Source: CAD feature listing. Evaluate the final solid. Frame: model axes, mm. Face numbers are marked on the shaded views. A direction names the side the tool comes from. Give positions to 0.01 mm unless a question says otherwise; leave off trailing zeros. Order: outer loops, then holes, each group sorted by start corner. A loop starts at its lowest first (then second) coordinate and runs counter-clockwise, first axis right, second up. Notation, with made-up numbers: (31.25, 13) -> (75.25, 13) arc R14 cw to (75.25, 24) -> close; hole circle Ø3 at (-35, 43.25). An arc over 180 degrees is marked (long way). Answer in a Markdown table with one row per item.
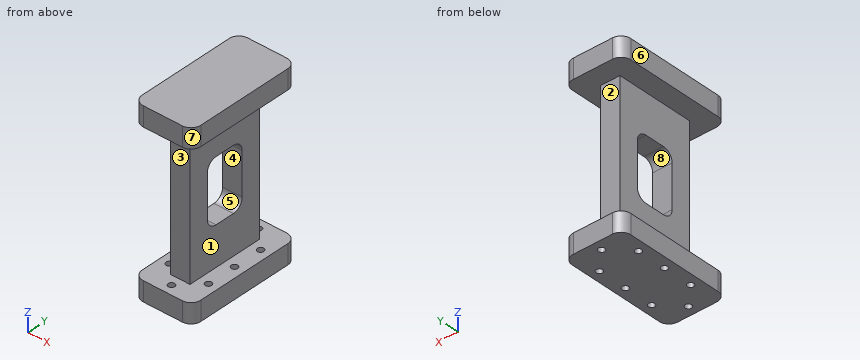
```python
from build123d import *

# Parameters (mm, degrees)
BOSS_EXTRUDE1_DEPTH       = 92
CUT_EXTRUDE1_DEPTH        = 102.311401135
CUT_EXTRUDE1_DEPTH_BACK   = 10
SKETCH3_W                 = 72
SKETCH3_H                 = 50
CUT_EXTRUDE2_DEPTH        = 10
SKETCH4_W                 = 72
SKETCH4_H                 = 10
CUT_EXTRUDE3_DEPTH        = 10
SKETCH5_W                 = 72
SKETCH5_H                 = 10
CUT_EXTRUDE4_DEPTH        = 10
M4X0_7_TAPPED_HOLE1_D     = 3.3
M4X0_7_TAPPED_HOLE1_DEPTH = 10
M4X0_7_TAPPED_HOLE2_D     = 3.3
M4X0_7_TAPPED_HOLE2_DEPTH = 10
M4X0_7_TAPPED_HOLE3_D     = 3.3
M4X0_7_TAPPED_HOLE3_DEPTH = 10
M4X0_7_TAPPED_HOLE4_D     = 3.3
M4X0_7_TAPPED_HOLE4_DEPTH = 10
M4X0_7_TAPPED_HOLE5_D     = 3.3
M4X0_7_TAPPED_HOLE5_DEPTH = 10
M4X0_7_TAPPED_HOLE6_D     = 3.3
M4X0_7_TAPPED_HOLE6_DEPTH = 10
M4X0_7_TAPPED_HOLE7_D     = 3.3
M4X0_7_TAPPED_HOLE7_DEPTH = 10
M4X0_7_TAPPED_HOLE8_D     = 3.3
M4X0_7_TAPPED_HOLE8_DEPTH = 10
CUT_EXTRUDE5_DEPTH        = 10
CUT_EXTRUDE8_DEPTH        = 10
CUT_EXTRUDE9_DEPTH        = 10


with BuildPart() as part:
    # Sketch1 → Boss-Extrude1 (new body)
    with BuildSketch(Plane.XY):
        with BuildLine():
            Line((-10, -30), (10, -30))
            ThreePointArc((10, -30), (13.535533906, -28.535533906), (15, -25))
            Line((15, -25), (15, 25))
            ThreePointArc((15, 25), (13.535533906, 28.535533906), (10, 30))
            Line((10, 30), (-10, 30))
            ThreePointArc((-10, 30), (-13.535533906, 28.535533906), (-15, 25))
            Line((-15, 25), (-15, -25))
            ThreePointArc((-15, -25), (-13.535533906, -28.535533906), (-10, -30))
        make_face()
    extrude(amount=BOSS_EXTRUDE1_DEPTH)

    # Sketch2 → Cut-Extrude1 (cut, two sides: drawn at the far end of the back side and taken through both)
    with BuildSketch(Plane(origin=(15, 0, 0), x_dir=(0, 0, -1), z_dir=(1, 0, 0)).offset(-CUT_EXTRUDE1_DEPTH_BACK)):
        Polygon((-10, 25), (-82, 25), (-82, -25), (-10, -25), (-10, 0), align=None)
    extrude(amount=CUT_EXTRUDE1_DEPTH + CUT_EXTRUDE1_DEPTH_BACK, mode=Mode.SUBTRACT)

    # Sketch3 → Cut-Extrude2 (cut)
    with BuildSketch(Plane.ZY.offset(15)):
        with Locations((46, 0)):
            Rectangle(SKETCH3_W, SKETCH3_H)
    extrude(amount=-CUT_EXTRUDE2_DEPTH, mode=Mode.SUBTRACT)

    # Sketch4 → Cut-Extrude3 (cut)
    with BuildSketch(Plane.ZY.offset(5)):
        with Locations((46, 25)):
            Rectangle(SKETCH4_W, SKETCH4_H)
    extrude(amount=-CUT_EXTRUDE3_DEPTH, mode=Mode.SUBTRACT)

    # Sketch5 → Cut-Extrude4 (cut)
    with BuildSketch(Plane.ZY.offset(5)):
        with Locations((46, -25)):
            Rectangle(SKETCH5_W, SKETCH5_H)
    extrude(amount=-CUT_EXTRUDE4_DEPTH, mode=Mode.SUBTRACT)

    # M4x0.7 Tapped Hole1
    with Locations(Plane.XY.offset(10)):
        with Locations((10, -15)):
            Hole(M4X0_7_TAPPED_HOLE1_D / 2, depth=M4X0_7_TAPPED_HOLE1_DEPTH)

    # M4x0.7 Tapped Hole2
    with Locations(Plane.XY.offset(10)):
        with Locations((10, 0)):
            Hole(M4X0_7_TAPPED_HOLE2_D / 2, depth=M4X0_7_TAPPED_HOLE2_DEPTH)

    # M4x0.7 Tapped Hole3
    with Locations(Plane.XY.offset(10)):
        with Locations((10, 15)):
            Hole(M4X0_7_TAPPED_HOLE3_D / 2, depth=M4X0_7_TAPPED_HOLE3_DEPTH)

    # M4x0.7 Tapped Hole4
    with Locations(Plane.XY.offset(10)):
        with Locations((-10, -15)):
            Hole(M4X0_7_TAPPED_HOLE4_D / 2, depth=M4X0_7_TAPPED_HOLE4_DEPTH)

    # M4x0.7 Tapped Hole5
    with Locations(Plane.XY.offset(10)):
        with Locations((-10, 0)):
            Hole(M4X0_7_TAPPED_HOLE5_D / 2, depth=M4X0_7_TAPPED_HOLE5_DEPTH)

    # M4x0.7 Tapped Hole6
    with Locations(Plane.XY.offset(10)):
        with Locations((-10, 15)):
            Hole(M4X0_7_TAPPED_HOLE6_D / 2, depth=M4X0_7_TAPPED_HOLE6_DEPTH)

    # M4x0.7 Tapped Hole7
    with Locations(Plane.XY.offset(10)):
        with Locations((0, 25)):
            Hole(M4X0_7_TAPPED_HOLE7_D / 2, depth=M4X0_7_TAPPED_HOLE7_DEPTH)

    # M4x0.7 Tapped Hole8
    with Locations(Plane.XY.offset(10)):
        with Locations((0, -25)):
            Hole(M4X0_7_TAPPED_HOLE8_D / 2, depth=M4X0_7_TAPPED_HOLE8_DEPTH)

    # Sketch27 → Cut-Extrude5 (cut)
    with BuildSketch(Plane.ZY.offset(5)):
        with BuildLine():
            Line((62, 0), (62, 5))
            ThreePointArc((62, 5), (60.535533906, 8.535533906), (57, 10))
            Line((57, 10), (35, 10))
            ThreePointArc((35, 10), (31.464466094, 8.535533906), (30, 5))
            Line((30, 5), (30, 0))
            Line((30, 0), (30, -5))
            ThreePointArc((30, -5), (31.464466094, -8.535533906), (35, -10))
            Line((35, -10), (57, -10))
            ThreePointArc((57, -10), (60.535533906, -8.535533906), (62, -5))
            Line((62, -5), (62, 0))
        make_face()
    extrude(amount=-CUT_EXTRUDE5_DEPTH, mode=Mode.SUBTRACT)

    # Sketch29 → Cut-Extrude8 (cut)
    with BuildSketch(Plane.ZY.offset(15)):
        Polygon((82, -25), (82, 25), (82, 39.435498448), (10, 39.435498448), (10, -37.130826461), (82, -37.130826461), align=None)
    extrude(amount=-CUT_EXTRUDE8_DEPTH, mode=Mode.SUBTRACT)

    # Sketch30 → Cut-Extrude9 (cut)
    with BuildSketch(Plane(origin=(15, 0, 0), x_dir=(0, 0, -1), z_dir=(1, 0, 0))):
        Polygon((-82, 25), (-82, -25), (-82, -44.187859425), (-10, -44.187859425), (-10, -25), (-10, 35.921267628), (-82, 35.921267628), align=None)
    extrude(amount=-CUT_EXTRUDE9_DEPTH, mode=Mode.SUBTRACT)


solid = part.part
```
(1) Pull-direction query (Y, two-part tool) for the marked faces 5, 6, 7 and 8; classes: +Y half, -Y half, draft (parallel to the pull), parting line (faces both ways), or undercut.
A:
| item | result |
|---|---|
| face 5 | undercut |
| face 6 | draft |
| face 7 | -Y half |
| face 8 | undercut |
(2) First-contact query: pin 1 Ø11 at (x, z) = (-2, 37.5) entering from -Y; pin 2 Ø10 at (x, z) = (-7.5, 31.5) entering from +Y; pin 3 Ø2.5 at (x, y) = (10, 0) entering from -Z; pin 4 Ø1.5 at (x, z) = (-6, 12.5) entering from +Y. Flat tips, straight axial feed; report the tip coordinate or a pass-through.
A:
| item | result |
|---|---|
| pin 1 | stops at y = -20 |
| pin 2 | stops at y = 20 |
| pin 3 | stops at z = 82 |
| pin 4 | passes through |
(3) Section query B-B (z = 42.5). Return the cut outline in (x, y), plus the area to 3 significant figures.
A:
| item | result |
|---|---|
| outline | (-5, -20) -> (5, -20) -> (5, -10) -> (-5, -10) -> close; (-5, 10) -> (5, 10) -> (5, 20) -> (-5, 20) -> close |
| area | 200 mm^2 |
(4) Section query A-A (y = 0). Return the cut outline in (x, z).
A:
| item | result |
|---|---|
| outline | (-15, 0) -> (-11.65, 0) -> (-11.65, 10) -> (-15, 10) -> close; (-15, 82) -> (-5, 82) -> (-5, 62) -> (5, 62) -> (5, 82) -> (15, 82) -> (15, 92) -> (-15, 92) -> close; (-8.35, 0) -> (8.35, 0) -> (8.35, 10) -> (5, 10) -> (5, 30) -> (-5, 30) -> (-5, 10) -> (-8.35, 10) -> close; (11.65, 0) -> (15, 0) -> (15, 10) -> (11.65, 10) -> close |
(5) Section query D-D (y = 15). Return the cut outline in (x, z), plus the area to 3 significant figures.
A:
| item | result |
|---|---|
| outline | (-15, 0) -> (-11.65, 0) -> (-11.65, 10) -> (-15, 10) -> close; (-15, 82) -> (-5, 82) -> (-5, 10) -> (-8.35, 10) -> (-8.35, 0) -> (8.35, 0) -> (8.35, 10) -> (5, 10) -> (5, 82) -> (15, 82) -> (15, 92) -> (-15, 92) -> close; (11.65, 0) -> (15, 0) -> (15, 10) -> (11.65, 10) -> close |
| area | 1,250 mm^2 |
(6) Access query for the marked faces 1, 2, 3 and 4. Directions: +Z, -Z, +X, -X, +Y, -Y. A direction counts if a zero-diameter tool reaches every point of the face in a straight line with its end or side. Return the directions, or none.
A:
| item | result |
|---|---|
| face 1 | +X, +Y, -Y |
| face 2 | +X, -X, +Y |
| face 3 | +X, -X, -Y |
| face 4 | +X, -X |
(7) Section query C-C (x = -0.25). Return the cut outline in (y, z), plus the area to 3 significant figures.
A:
| item | result |
|---|---|
| outline | (-30, 0) -> (-26.63, 0) -> (-26.63, 10) -> (-30, 10) -> close; (-30, 82) -> (-20, 82) -> (-20, 10) -> (-23.37, 10) -> (-23.37, 0) -> (23.37, 0) -> (23.37, 10) -> (20, 10) -> (20, 82) -> (30, 82) -> (30, 92) -> (-30, 92) -> close; (26.63, 0) -> (30, 0) -> (30, 10) -> (26.63, 10) -> close; hole (-10, 35) arc R5 ccw to (-5, 30) -> (5, 30) arc R5 ccw to (10, 35) -> (10, 57) arc R5 ccw to (5, 62) -> (-5, 62) arc R5 ccw to (-10, 57) -> close |
| area | 3,400 mm^2 |
(8) Ray query, probe 1 along Y at (x, z) = (-10, 7.25); probe 2 along Z at (x, y) = (9.5, 24); probe 3 along Y at (x, z) = (0, 6.75). Return the intervals inside material, ascending.
A:
| item | result |
|---|---|
| probe 1 | y = -30 to -16.65, -13.35 to -1.65, 1.65 to 13.35, 16.65 to 30 |
| probe 2 | z = 0 to 10, 82 to 92 |
| probe 3 | y = -30 to -26.65, -23.35 to 23.35, 26.65 to 30 |
